```python
from build123d import *

# Parameters (mm, degrees)
F0_W      = 48
F0_H      = 50
F1_DEPTH  = 48
F2_W      = 6
F2_H      = 10
F3_DEPTH  = 96.001
F4_W      = 19
F4_H      = 24
F5_DEPTH  = 16
F7_DEPTH  = 29.001
F9_DEPTH  = 48.001
F10_W     = 19
F10_H     = 24
F11_DEPTH = 16
F13_DEPTH = 29.001


with BuildPart() as f1:
    # F0 (on Front) → F1 (new body, symmetric)
    with BuildSketch(Plane.XZ):
        Rectangle(F0_W, F0_H)
    extrude(amount=F1_DEPTH, both=True)

    # F2 (on face) → F3 (cut, through all)
    with BuildSketch(Plane.XZ.offset(48)):
        with Locations((-21, -20)):
            Rectangle(F2_W, F2_H)
        with Locations((21, -20)):
            Rectangle(F2_W, F2_H)
    extrude(amount=-F3_DEPTH, mode=Mode.SUBTRACT)

    # F4 (on face) → F5 (cut)
    with BuildSketch(Plane.XZ.offset(48)):
        with Locations((-14.5, 13)):
            Rectangle(F4_W, F4_H)
        with Locations((14.5, 13)):
            Rectangle(F4_W, F4_H)
    extrude(amount=-F5_DEPTH, mode=Mode.SUBTRACT)

    # F6 (on face) → F7 (cut, through all)
    with BuildSketch(Plane(origin=(-5, 0, 0), x_dir=(0, -1, 0), z_dir=(-1, 0, 0))):
        Polygon((32, 17), (48, 1), (48, 25), (32, 25), align=None)
    extrude(amount=-F7_DEPTH, mode=Mode.SUBTRACT)

    # F8 (on face) → F9 (cut, through all)
    with BuildSketch(Plane(origin=(-24, 0, 0), x_dir=(0, -1, 0), z_dir=(-1, 0, 0))):
        Polygon((12, 15), (22, 25), (-22, 25), (-12, 15), (-12, 9), (12, 9), align=None)
    extrude(amount=-F9_DEPTH, mode=Mode.SUBTRACT)

    # F10 (on face) → F11 (cut)
    with BuildSketch(Plane(origin=(0, 48, 0), x_dir=(-1, 0, 0), z_dir=(0, 1, 0))):
        with Locations((-14.5, 13)):
            Rectangle(F10_W, F10_H)
        with Locations((14.5, 13)):
            Rectangle(F10_W, F10_H)
    extrude(amount=-F11_DEPTH, mode=Mode.SUBTRACT)

    # F12 (on face) → F13 (cut, through all)
    with BuildSketch(Plane(origin=(-5, 0, 0), x_dir=(0, -1, 0), z_dir=(-1, 0, 0))):
        Polygon((-48, 1), (-32, 17), (-32, 25), (-48, 25), align=None)
    extrude(amount=-F13_DEPTH, mode=Mode.SUBTRACT)


solid = f1.part
```
Can you work these out from the model? Positions are in its coordinate system, mm. A direction names the side the tool comes from. Give positions to 0.01 mm unless a question says otherwise; leave off trailing zeros. Order: outer loops, then holes, each group sorted by start corner. A loop starts at its lowest first (then second) coordinate and runs counter-clockwise, first axis right, second up. Notation, with made-up numbers: M 83.5,36.25 L 124.5,36.25 A16 cw 124.5,59.25 Z; hole C 4.25,21 d3. An arc over 180 degrees is marked long. One line per item, written item: value.
1) I want a section at C-C, the plane z = 6.5. List the corners of the cut face in (x, y) for me.
Answer sheet:
outline: M -24,-32 L -5,-32 L -5,-42.5 L 5,-42.5 L 5,-32 L 24,-32 L 24,32 L 5,32 L 5,42.5 L -5,42.5 L -5,32 L -24,32 Z
2) I want a section at B-B, the plane x = -14. List the corners of the cut face in (y, z) for me, plus the area to 3 significant figures.
Answer sheet:
outline: M -48,-25 L 48,-25 L 48,1 L 32,1 L 32,25 L 22,25 L 12,15 L 12,9 L -12,9 L -12,15 L -22,25 L -32,25 L -32,1 L -48,1 Z
area: 3,550 mm^2
3) I want a section at A-A, the plane y = -41. List the corners of the cut face in (x, z) for me, plus the area to 3 significant figures.
Answer sheet:
outline: M -24,-15 L -18,-15 L -18,-25 L 18,-25 L 18,-15 L 24,-15 L 24,1 L 5,1 L 5,8 L -5,8 L -5,1 L -24,1 Z
area: 1,200 mm^2
4) On a 3-axis mill with a long thin cutter (end or side, diameter ignored), from which of +Z, -Z, +X, -X, +Y, -Y can I reach the whole of each face in a straight line? I mean faces 1 (the face through (0, 12, 12)), 2 (the face through (-18, -1, -20)), 3 (the face through (18, -1, -20)), 4 (the face through (5, -37, 5)), 5 (the face through (5, 37, 5)). Say none if no direction works.
Answer sheet:
face 1: +Z, +X, -X
face 2: -Z, -X, +Y, -Y
face 3: -Z, +X, +Y, -Y
face 4: +Z, +X, -Y
face 5: +Z, +X, +Y
5) I want a section at D-D, the plane y = 28.5. List the corners of the cut face in (x, z) for me.
Answer sheet:
outline: M -24,-15 L -18,-15 L -18,-25 L 18,-25 L 18,-15 L 24,-15 L 24,25 L -24,25 Z
6) Please list where these lines run through material, in increasing order: line 1 along Y through (x, z) = (-13.5, 13); line 2 along Z through (x, y) = (20, -3.5); line 3 along Z through (x, y) = (-19.5, 39).
Answer sheet:
line 1: y = -32 to -12, 12 to 32
line 2: z = -15 to 9
line 3: z = -15 to 1
7) We'd pull the mould along Y, two halves only. Please class faces 6 (the face through (0, 17, 20)), 7 (the face through (14, -40, 1)), 8 (the face through (0, -48, -12)): released by +Y, released by -Y, zero draft, split by the parting line, or undercut.
Answer sheet:
face 6: undercut
face 7: zero draft
face 8: released by -Y
8) For P1, Ø8, axis at x = 1.5, z = 14.5, coming from the -Y side; P2, Ø5, axis at x = -21, y = 22, coming from the -Z side; P3, Ø19, axis at x = -1.5, z = 13, coming from the +Y side, each with a flat end and sliding along its axis, tell me the tip position at first contact or that it passes through.
Answer sheet:
P1: stops at y = -38.5
P2: stops at z = -15
P3: stops at y = 45.5
